Read the model definition and answer for the solid it produces. Units are mm, in the model's axes. A direction names the side the tool comes from. Round coordinates to 2 decimals unless told otherwise and drop trailing zeros. Order: outer loops, then holes, each group sorted by start corner. A loop starts at its lowest first (then second) coordinate and runs counter-clockwise, first axis right, second up. Notation, with made-up numbers: (-21.5, -26) - (18.5, -26) arc R19 ccw to (18.5, -14) - close; hole circle Ø2 at (-20, 1.25). An arc over 180 degrees is marked (long way). One line per question, with ' | ' between items. Start each with the question number.
1) The part is cut by section A-A, the plane z = 9.5. Give the vertices of the cut face in (x, y).
2) The part is cut by section D-D, the plane x = 85. Give the vertices of the cut face in (y, z), plus the area to 3 significant figures.
3) Straight lines are drawn through the part: line 1 (X direction, y = -14, z = 13.5); line 2 (X direction, y = -6.5, z = 9.5); line 3 (Y direction, x = 65.25, z = 9.5). For each, find the intervals that lie inside material, in ascending order. Write a range as from..to.
4) Flat-ended cylindrical pins translate along their axes: pin 1 (3 mm diameter, centred on y = -22.94, z = 9.5, fed in from +X); pin 2 (5.5 mm diameter, centred on y = -22, z = 10.5, fed in from +X); pin 3 (5 mm diameter, centred on y = -22.94, z = 9.5, fed in from -X); pin 4 (4.5 mm diameter, centred on x = 85, z = 9.5, fed in from -Y). Find the tip coordinate at first contact, or state that the pin passes through.
5) For faces 1 (the flat face through (69, -23, 12)), 2 (the flat face through (80, -19, 9)), 3 (the flat face through (60, -19, 9)), determine the directions among +Z, -Z, +X, -X, +Y, -Y from which every point of the face is accessible in a straight line to the end or side of a thin tool.
6) The part is cut by section C-C, the plane x = 72. Give the vertices of the cut face in (y, z), plus the area to 3 significant figures.
7) The mould has two halves that part along Y. Classify faces 4 (the cylindrical face through (75.56, -24.89, 9.07)), 5 (the cylindrical face through (70, -10, 9)), 6 (the flat face through (70, 0, 9)), 7 (the flat face through (55, -10, 7)): pulls with the +Y half, pulls with the -Y half, needs draft (parallel to the pull), parting line crosses it, or undercut.
8) The part is cut by section B-B, the plane y = -14. Give the vertices of the cut face in (x, z).
from build123d import *

# Parameters (mm, degrees)
SKETCH1_R               = 4
BOSS_EXTRUDE1_DEPTH     = 19
SKETCH3_R               = 2
CUT_EXTRUDE2_DEPTH      = 10
SKETCH4_W               = 2
SKETCH4_H               = 25.552295944
CUT_EXTRUDE3_DEPTH      = 19
CUT_EXTRUDE4_DEPTH      = 40.824615503
CUT_EXTRUDE4_DEPTH_BACK = 40.824615503
SKETCH5_R               = 2


with BuildPart() as part:
    # Sketch1 → Boss-Extrude1 (new body)
    with BuildSketch(Plane.XY):
        Polygon((50, 0), (90, 0), (90, -10), (80, -10), (80, -28), (60, -28), (60, -10), (50, -10), align=None)
        with Locations((70, -14)):
            Circle(SKETCH1_R, mode=Mode.SUBTRACT)
    extrude(amount=BOSS_EXTRUDE1_DEPTH)

    # Sketch3 → Cut-Extrude2 (cut)
    with BuildSketch(Plane(origin=(0, -10, 0), x_dir=(-1, 0, 0), z_dir=(0, -1, 0))):
        with Locations(Location((-85, -9.5, 0), (0, 0, 90))):
            Circle(SKETCH3_R)
        with Locations(Location((-55, -9.5, 0), (0, 0, 90))):
            Circle(SKETCH3_R)
    extrude(amount=-CUT_EXTRUDE2_DEPTH, mode=Mode.SUBTRACT)

    # Sketch4 → Cut-Extrude3 (cut)
    with BuildSketch(Plane.XY.offset(19)):
        with Locations((70, -28)):
            Rectangle(SKETCH4_W, SKETCH4_H)
    extrude(amount=-CUT_EXTRUDE3_DEPTH, mode=Mode.SUBTRACT)

    # Sketch5 → Cut-Extrude4 (cut, two sides: drawn at the far end of the back side and taken through both)
    with BuildSketch(Plane.ZY.offset(-71).offset(-CUT_EXTRUDE4_DEPTH_BACK)):
        with Locations((9.5, -22.936491673)):
            Circle(SKETCH5_R)
    extrude(amount=CUT_EXTRUDE4_DEPTH + CUT_EXTRUDE4_DEPTH_BACK, mode=Mode.SUBTRACT)


solid = part.part
Values:
1) outline: (50, -10) - (53, -10) - (53, 0) - (50, 0) - close; (57, -10) - (60, -10) - (60, -20.94) - (69, -20.94) - (69, -17.87) arc R4 cw (long way) to (71, -17.87) - (71, -20.94) - (80, -20.94) - (80, -10) - (83, -10) - (83, 0) - (57, 0) - close; (60, -28) - (69, -28) - (69, -24.94) - (60, -24.94) - close; (71, -28) - (80, -28) - (80, -24.94) - (71, -24.94) - close; (87, -10) - (90, -10) - (90, 0) - (87, 0) - close
2) outline: (-10, 0) - (0, 0) - (0, 7.5) - (-10, 7.5) - close; (-10, 11.5) - (0, 11.5) - (0, 19) - (-10, 19) - close | area: 150 mm^2
3) line 1: x = 60..66, 74..80 | line 2: x = 50..53, 57..83, 87..90 | line 3: y = -28..-24.94, -20.94..0
4) pin 1: passes through | pin 2: stops at x = 80 | pin 3: stops at x = 60 | pin 4: stops at y = -10
5) face 1: +Z, -Z, -Y | face 2: +Z, -Z, +X, -Y | face 3: +Z, -Z, -X, -Y
6) outline: (-28, 0) - (-17.46, 0) - (-17.46, 19) - (-28, 19) - close; (-10.54, 0) - (0, 0) - (0, 19) - (-10.54, 19) - close; hole circle Ø4 at (-22.94, 9.5) | area: 388 mm^2
7) face 4: undercut | face 5: undercut | face 6: pulls with the +Y half | face 7: pulls with the -Y half
8) outline: (60, 0) - (66, 0) - (66, 19) - (60, 19) - close; (74, 0) - (80, 0) - (80, 19) - (74, 19) - close
